The listing builds one solid part. Answer for the finished solid, in the listing's coordinates (mm). A direction names the side the tool comes from. Round coordinates to 2 decimals unless told otherwise and drop trailing zeros. Order: outer loops, then holes, each group sorted by start corner. A loop starts at its lowest first (then second) coordinate and runs counter-clockwise, first axis right, second up. Notation, with made-up numbers: M -36,70 L -30,70 A35 cw -30,104 Z; hole C -3.75,43.25 d2. An arc over 180 degrees is marked long. Write item = value, one per line. Start each with the question number.
(1) A cutting plane is placed at A-A, the plane z = -1. Determine the outline of the cut face in (x, y).
(2) A cutting plane is placed at B-B, the plane z = -6. Determine the outline of the cut face in (x, y).
(3) Each of these flat-tipped pins is pushed along its axis until it touches: pin 1 (1 mm diameter, centred on x = 2.5, y = 7.5, fed in from -Z); pin 2 (1.6 mm diameter, centred on x = 6, z = 5.5, fed in from -Y); pin 3 (2 mm diameter, centred on y = 6, z = 0.5, fed in from +X). Where does it stop, or does it pass through?
(4) A cutting plane is placed at C-C, the plane y = 14. Determine the outline of the cut face in (x, z), and give its area (3 significant figures).
(5) Which of the six approach directions +Z, -Z, +X, -X, +Y, -Y give full straight-line access (tool end or side, diameter ignored) to faces 1 (the face through (4.46, 9.23, 24.45)), 2 (the face through (4.465, -21.785, 14.342)), 3 (the face through (6, 2, 5))?
(6) Straight lines are drawn through the part: probe 1 along Z at (x, y) = (3.4, -24); probe 2 along Y at (x, z) = (6.1, 24.5); probe 3 along Y at (x, z) = (6.3, 19). For each, find the intervals that lie inside material, in ascending order. Write a range as from..to.
from build123d import *

# Parameters (mm, degrees)
BASPROSKE_W             = 7
BASPROSKE_H             = 27.75
TOOTHCUT_DEPTH          = 40.863830724
TEETHCUTS_COUNT         = 35
TEETHCUTS_ANGLE         = 349.714285714
BORSKE_R                = 3
BORE_DEPTH              = 50.0000508
CUT_EXTRUDE1_DEPTH      = 2
CUT_EXTRUDE2_DEPTH      = 2
CUT_EXTRUDE3_DEPTH      = 10
CUT_EXTRUDE4_DEPTH      = 2
FILLET2_R               = 5
CUT_EXTRUDE5_DEPTH      = 10
FILLET3_R               = 5
CUT_EXTRUDE6_DEPTH      = 40.804405632
CUT_EXTRUDE6_DEPTH_BACK = 40.804405632


with BuildPart() as part:
    # BasProSke → Base-Revolve (revolve)
    with BuildSketch(Plane(origin=(0, 0, 0), x_dir=(1, 0, 0), z_dir=(0, 1, 0)), mode=Mode.PRIVATE) as base_revolve_sk:
        with Locations((3.5, 13.875)):
            Rectangle(BASPROSKE_W, BASPROSKE_H)
    revolve(base_revolve_sk.sketch.rotate(Axis((-10, 0, 0), (1, 0, 0)), 180), axis=Axis((-10, 0, 0), (1, 0, 0)))

    # TooCutSke → ToothCut (cut, through all)
    with BuildSketch(Plane(origin=(0, 0, 0), x_dir=(0, 0, -1), z_dir=(1, 0, 0))):
        with BuildLine():
            ThreePointArc((0.678148312, 24.364564245), (0, 24.374), (-0.678148312, 24.364564245))
            ThreePointArc((-0.678148312, 24.364564245), (-1.217075524, 26.091376176), (-2.044396801, 27.70005933))
            ThreePointArc((-2.044396801, 27.70005933), (0, 27.7754), (2.044396801, 27.70005933))
            ThreePointArc((2.044396801, 27.70005933), (1.217075524, 26.091376176), (0.678148312, 24.364564245))
        make_face()
    toothcut = extrude(amount=TOOTHCUT_DEPTH, mode=Mode.SUBTRACT)

    # TeethCuts: ToothCut ×35 about axis
    teethcuts_axis = Axis((-10, 0, 0), (1, 0, 0))
    for i in range(1, TEETHCUTS_COUNT):
        add(toothcut.rotate(teethcuts_axis, i * TEETHCUTS_ANGLE / (TEETHCUTS_COUNT - 1)), mode=Mode.SUBTRACT)

    # BorSke → Bore (cut, symmetric)
    with BuildSketch(Plane(origin=(0, 0, 0), x_dir=(0, 0, -1), z_dir=(1, 0, 0))):
        with Locations(Location((0, 0, 0), (0, 0, 180))):
            Circle(BORSKE_R)
    extrude(amount=BORE_DEPTH, both=True, mode=Mode.SUBTRACT)

    # Sketch3 → Cut-Extrude1 (cut)
    with BuildSketch(Plane(origin=(7, 0, 0), x_dir=(0, 0, -1), z_dir=(1, 0, 0))):
        with BuildLine():
            Line((-1.5, -7.5), (-1.5, 7.5))
            ThreePointArc((-1.5, 7.5), (0, 9), (1.5, 7.5))
            Line((1.5, 7.5), (1.5, -7.5))
            ThreePointArc((1.5, -7.5), (0, -9), (-1.5, -7.5))
        make_face()
    extrude(amount=-CUT_EXTRUDE1_DEPTH, mode=Mode.SUBTRACT)

    # Sketch4 → Cut-Extrude2 (cut)
    with BuildSketch(Plane(origin=(7, 0, 0), x_dir=(0, 0, -1), z_dir=(1, 0, 0))):
        with BuildLine():
            Line((-7.5, 1.5), (7.5, 1.5))
            ThreePointArc((7.5, 1.5), (9, 0), (7.5, -1.5))
            Line((7.5, -1.5), (-7.5, -1.5))
            ThreePointArc((-7.5, -1.5), (-9, 0), (-7.5, 1.5))
        make_face()
    extrude(amount=-CUT_EXTRUDE2_DEPTH, mode=Mode.SUBTRACT)

    # Sketch5 → Cut-Extrude3 (cut)
    with BuildSketch(Plane(origin=(7, 0, 0), x_dir=(0, 0, -1), z_dir=(1, 0, 0))):
        with BuildLine():
            ThreePointArc((12.297844577, 0), (8.695889295, -8.695889295), (0, -12.297844577))
            Line((0, -12.297844577), (0, -32.483772695))
            ThreePointArc((0, -32.483772695), (32.823056407, 0.339283713), (0, 33.16234012))
            Line((0, 33.16234012), (0, 12.297844577))
            ThreePointArc((0, 12.297844577), (8.695889295, 8.695889295), (12.297844577, 0))
        make_face()
    extrude(amount=-CUT_EXTRUDE3_DEPTH, mode=Mode.SUBTRACT)

    # Sketch6 → Cut-Extrude4 (cut)
    with BuildSketch(Plane(origin=(7, 0, 0), x_dir=(0, 0, -1), z_dir=(1, 0, 0))):
        with BuildLine():
            Line((-2, 2), (-2, 7.5))
            ThreePointArc((-2, 7.5), (0, 9.5), (2, 7.5))
            Line((2, 7.5), (2, 2))
            Line((2, 2), (7.5, 2))
            ThreePointArc((7.5, 2), (9.5, 0), (7.5, -2))
            Line((7.5, -2), (2, -2))
            Line((2, -2), (2, -7.5))
            ThreePointArc((2, -7.5), (0, -9.5), (-2, -7.5))
            Line((-2, -7.5), (-2, -2))
            Line((-2, -2), (-7.5, -2))
            ThreePointArc((-7.5, -2), (-9.5, 0), (-7.5, 2))
            Line((-7.5, 2), (-2, 2))
        make_face()
    extrude(amount=-CUT_EXTRUDE4_DEPTH, mode=Mode.SUBTRACT)

    # Fillet2
    fillet2_edges = [part.edges().sort_by_distance(p)[0] for p in [
        (3.5, -12.297844577, 0),
        (3.5, 12.297844577, 0),
    ]]
    fillet(fillet2_edges, radius=FILLET2_R)

    # Sketch8 → Cut-Extrude5 (cut)
    with BuildSketch(Plane(origin=(7, 0, 0), x_dir=(0, 0, -1), z_dir=(1, 0, 0))):
        Polygon((-2.859440987, -24.205690927), (-1.508604415, -24.327268419), (1.243700079, -24.574980307), (1.243700079, -32.134713867), (-1.933875746, -26.979191879), align=None)
    extrude(amount=-CUT_EXTRUDE5_DEPTH, mode=Mode.SUBTRACT)

    # Fillet3
    # the kernel refuses this fillet: 5 mm, written as the material it takes off along each edge
    with BuildSketch(Plane(origin=(13.309286436, 24.374, 0), x_dir=(0, -1, 0), z_dir=(-1, 0, 0))) as fillet3_piece_1:
        with BuildLine():
            CenterArc((2.523714574, 5), FILLET3_R, 239.81088364, 30.18911636)
            Line((0.009435755, 0.678148312), (-0.040849822, 0.591711278))
            ThreePointArc((-0.040849822, 0.591711278), (-0.097631269, 0.340498242), (-0.1, 0))
            Line((-0.1, 0), (0, -0.1))
            Line((0, -0.1), (2.523714574, -0.1))
            Line((2.523714574, -0.1), (2.523714574, 0))
        make_face()
    extrude(amount=19.618572871, mode=Mode.SUBTRACT)
    with BuildSketch(Plane(origin=(-11.93995811, -24.463045274, 0), x_dir=(0, 0.08963930890343594, 0.995974293995239), z_dir=(1, 0, 0))) as fillet3_piece_2:
        with BuildLine():
            CenterArc((5.407987307, -4.308559995), FILLET3_R, 120.490647096, 64.652210046)
            Line((0.428115837, -4.75675654), (0.328518408, -4.76572047))
            Line((0.328518408, -4.76572047), (-0.099597429, -0.008963931))
            Line((-0.099597429, -0.008963931), (0, 0.1))
            ThreePointArc((0, 0.1), (1.435499392, 0.1), (2.820259013, 0.0861712))
            Line((2.820259013, 0.0861712), (2.870998784, 0))
        make_face()
    extrude(amount=30.87991622, mode=Mode.SUBTRACT)

    # Sketch9 → Cut-Extrude6 (cut, two sides: drawn at the far end of the back side and taken through both)
    with BuildSketch(Plane(origin=(0, 0, 0), x_dir=(1, 0, 0), z_dir=(0, 1, 0)).offset(-CUT_EXTRUDE6_DEPTH_BACK)):
        Polygon((-2.448455727, -28.878486524), (2, -28.878486524), (2, 12.992603003), (-3.949809534, 12.992603003), (-3.949809534, -28.878486524), align=None)
    extrude(amount=CUT_EXTRUDE6_DEPTH + CUT_EXTRUDE6_DEPTH_BACK, mode=Mode.SUBTRACT)


solid = part.part
Reported:
q1.outline = M 2,-13.56 L 7,-13.56 L 7,-9.23 L 5,-9.23 L 5,-2.83 L 2,-2.83 Z; M 2,2.83 L 5,2.83 L 5,9.23 L 7,9.23 L 7,13.56 L 2,13.56 Z
q2.outline = M 2,-10.73 L 7,-10.73 L 7,-2 L 5,-2 L 5,2 L 7,2 L 7,10.73 L 2,10.73 Z
q3.pin_1 = -10.11
q3.pin_2 = -27.35
q3.pin_3 = 5
q4.outline = M 2,-0.7 L 7,-0.7 L 7,22.83 L 2,22.83 Z
q4.area = 118 mm²
q5.face_1 = +Z, +X, -X
q5.face_2 = +X, -X
q5.face_3 = +X
q6.probe_1 = 2.47..5.84, 7.54..10.22, 13.75..13.93
q6.probe_2 = -13.03..-12.53, -9.14..-6.56, -4.75..-1.82, -0.39..2.57, 4.12..6.93, 9.27..11.35
q6.probe_3 = -16.85..15.27, 16.21..19.25
